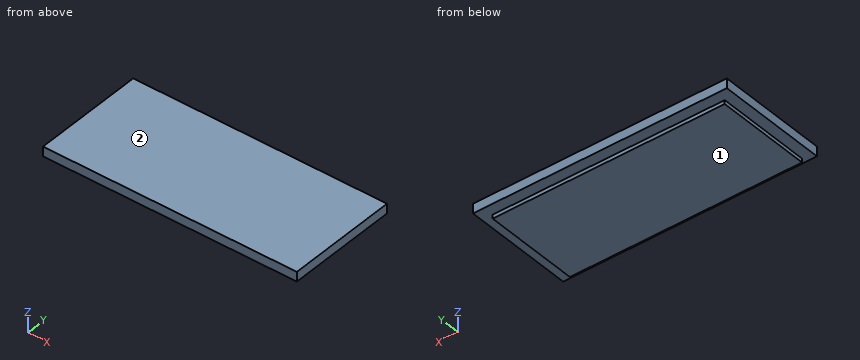
Autodesk Inventor part; units mm, degrees
ref_plane "YZ Plane" through (0, 0, 0) normal (1, 0, 0) x (0, 1, 0)
ref_plane "XZ Plane" through (0, 0, 0) normal (0, 1, 0) x (-1, 0, 0)
ref_plane "XY Plane" through (0, 0, 0) normal (0, 0, 1) x (1, 0, 0)
sketch "Skizze1" plane through (0, 0, 0) normal (0, 0, 1) x (1, 0, 0)
  line L0 (199, -87.5) -> (-199, -87.5)
  line L1 (-199, -87.5) -> (-199, 87.5)
  line L2 (-199, 87.5) -> (199, 87.5)
  line L3 (199, 87.5) -> (199, -87.5)
  line L4 (199, -87.5) -> (-199, 87.5) construction
  line L5 (-199, -87.5) -> (199, 87.5) construction
  line L6 (-182, 70.5) -> (182, 70.5)
  line L7 (182, 70.5) -> (182, -79.5)
  line L8 (182, -79.5) -> (-182, -79.5)
  line L9 (-182, -79.5) -> (-182, 70.5)
  line L10 (-182, 70.5) -> (182, -79.5) construction
  line L11 (182, 70.5) -> (-182, -79.5) construction
  point P0 (0, 0)
  point P1 (0, -4.5)
  point P2 (0, -4.5)
  point P3 (0, 0)
  dimension "d0" = 175
  dimension "d1" = 398
  dimension "d2" = 8
  dimension "d3" = 17
  dimension "d4" = 17
extrude "Extrusion1" add sketch "Skizze1" along normal blind 15 contours L0 L1 L2 L3 | L6 L7 L8 L9
extrude "Extrusion2" add sketch "Skizze1" against normal blind 6 contours L6 L7 L8 L9
equation "\"d1\" = case_width - 2 * gap_air"
equation "\"d5\" = inner_thickness"
equation "\"d7\" = mdf_thickness"
equation "\"kg_thickness\" = 4.9"
equation "\"ht_thickness\" = 1.9"
equation "\"case_thickness\" = 18"
equation "\"inner_thickness\" = 15"
equation "\"gap_fit\" = 0.1"
equation "\"gap_slide\" = 0.2"
equation "\"gap_air\" = 1"
equation "\"bore_diameter\" = 73"
equation "\"mdf_thickness\" = 6"
equation "\"tape_width\" = 15"
equation "\"tape_thickness\" = 3"
equation "\"inner_depth\" = 255"
properties part number "Front_Elektronik"
CAD build for the part. Positions are in the model's coordinates, mm. Face numbers are marked on the shaded views. Round coordinates to 2 decimals unless told otherwise and drop trailing zeros. Write each loop counter-clockwise with the first axis right and the second up, starting at its lowest first coordinate (ties: lowest second). Pieces come first, ordered by that corner, then holes. Notation, with made-up numbers: M 65.5,-19 L 116.5,-19 A15 cw 116.5,2 Z; hole C 11,59.25 d10. An arc over 180 degrees is marked long. Put each result on its own line as item: value. Start each with the question number.
1) Saw through at B-B, the plane x = 129. Write the cut outline in (y, z), and give its area (4 significant figures).
2) Drill centre lines: probe 1 along Y at (x, z) = (-64.5, -0.5); probe 2 along X at (y, z) = (-73.5, -4.75); probe 3 along Z at (x, y) = (-40.5, 77). Where is each one in solid material? Low to high. Write a range as [from, to].
3) Pull direction Z, two halves, no side cores. Call the marked faces 1 and 2: pulls with the +Z half, pulls with the -Z half, needs draft (parallel to the pull), parting line crosses it, or undercut.
4) Saw through at A-A, the plane y = -29. Write the cut outline in (x, z), and give its area (3 significant figures).
5) Pin check, flat tips, straight feed: pin 1 Ø10 at (y, z) = (-60.5, -2.5) entering from -X; pin 2 Ø1.8 at (y, z) = (-32.5, -4) entering from +X; pin 3 Ø6.5 at (x, z) = (-10.5, -4) entering from -Y. Stop position of each tip, or through.
Resolved:
1. outline: M -87.5,0 L -79.5,0 L -79.5,-6 L 70.5,-6 L 70.5,0 L 87.5,0 L 87.5,15 L -87.5,15 Z
1. area: 3,525 mm²
2. probe 1: [-79.5, 70.5]
2. probe 2: [-182, 182]
2. probe 3: [0, 15]
3. face 1: pulls with the -Z half
3. face 2: pulls with the +Z half
4. outline: M -199,0 L -182,0 L -182,-6 L 182,-6 L 182,0 L 199,0 L 199,15 L -199,15 Z
4. area: 8,150 mm²
5. pin 1: x = -199
5. pin 2: x = 182
5. pin 3: y = -79.5
